Part model, mm, in its own coordinate system. Give positions to 0.01 mm unless a question says otherwise; leave off trailing zeros. Write each loop counter-clockwise with the first axis right and the second up, starting at its lowest first coordinate (ties: lowest second). Pieces come first, ordered by that corner, then holes.
```python
from build123d import *

# Parameters (mm, degrees)
F1_DEPTH = 28
F3_DEPTH = 2503
F5_DEPTH = 28
F6_R     = 2
F7_R     = 1
F8_R     = 4.25
F9_DEPTH = 25


with BuildPart() as f1:
    # F0 (on Top) → F1 (new body)
    with BuildSketch(Plane.XY):
        Polygon((-19.75, -17.750001), (-19.75, -19.75), (-9.25, -19.75), (19.75, 9.25), (19.75, 19.75), (17.750001, 19.75), (17.750001, 10.078427), (-10.078427, -17.750001), align=None)
    extrude(amount=F1_DEPTH)

    # F2 (on face) → F3 (join)
    with BuildSketch(Plane.XY.offset(28)):
        Polygon((-19.75, -19.75), (-9.25, -19.75), (19.75, 9.25), (19.75, 19.75), (11.25, 19.75), (11.25, 24.25), (9.25, 26.25), (9.25, 23.421573), (9.25, 19.75), (9.25, 17.750001), (17.750001, 17.750001), (17.750001, 10.078427), (16.585787, 8.914213), (-8.914213, -16.585787), (-10.078427, -17.750001), (-17.750001, -17.750001), (-17.750001, -9.25), (-19.75, -9.25), (-23.421573, -9.25), (-26.25, -9.25), (-24.25, -11.25), (-19.75, -11.25), align=None)
    extrude(amount=F3_DEPTH)

    # F4 (on face) → F5 (join)
    with BuildSketch(Plane.XY.offset(2531)):
        Polygon((19.75, 9.25), (19.75, 19.75), (17.750001, 19.75), (17.750001, 10.078427), (-10.078427, -17.750001), (-19.75, -17.750001), (-19.75, -19.75), (-9.25, -19.75), align=None)
    extrude(amount=F5_DEPTH)

    # F6
    f6_edges = [f1.edges().sort_by_distance(p)[0] for p in [
        (19.75, 9.25, 1279.5),
        (-9.25, -19.75, 1279.5),
    ]]
    fillet(f6_edges, radius=F6_R)

    # F7
    f7_edges = [f1.edges().sort_by_distance(p)[0] for p in [
        (-19.75, -19.75, 1279.5),
        (19.75, 19.75, 1279.5),
    ]]
    fillet(f7_edges, radius=F7_R)

    # F8 (on face) → F9 (cut)
    with BuildSketch(Plane(origin=(5.25, -5.25, 0), x_dir=(0.707107, 0.707107, 0), z_dir=(0.707107, -0.707107, 0))):
        with Locations((0, 14)):
            Circle(F8_R)
    extrude(amount=-F9_DEPTH, mode=Mode.SUBTRACT)


solid = f1.part
```
1) Pin check, flat tips, straight feed: pin 1 Ø3 at (y, z) = (12.5, 890.5) entering from -X; pin 2 Ø9.5 at (x, z) = (12, 999) entering from -Y; pin 3 Ø4 at (y, z) = (23, 688.5) entering from -X. Stop position of each tip, or through.
Answers follow:
pin 1: stops at x = 17.75
pin 2: stops at y = -3.25
pin 3: stops at x = 9.25
2) Saw through at A-A, the plane z = 747. Write the cut outline in (x, y).
Answers follow:
outline: (-26.25, -9.25) - (-24.25, -11.25) - (-19.75, -11.25) - (-19.75, -18.75) arc R1 ccw to (-18.75, -19.75) - (-10.08, -19.75) arc R2 ccw to (-8.66, -19.16) - (19.16, 8.66) arc R2 ccw to (19.75, 10.08) - (19.75, 18.75) arc R1 ccw to (18.75, 19.75) - (11.25, 19.75) - (11.25, 24.25) - (9.25, 26.25) - (9.25, 17.75) - (17.75, 17.75) - (17.75, 10.08) - (-10.08, -17.75) - (-17.75, -17.75) - (-17.75, -9.25) - close
3) Wall check: L1, parallel to Y at x = -11, z = 1206; L2, parallel to X at y = 20, z = 225; L3, parallel to Y at x = -21.5, z = 1864.5. Give the ranges that are in metal, low to high.
Answers follow:
L1: y = -19.75 to -17.75
L2: x = 9.25 to 11.25
L3: y = -11.25 to -9.25
